Read the model definition and answer for the solid it produces. Units are mm, in the model's axes. A direction names the side the tool comes from. Coordinates: 2 decimals unless noted, no trailing zeros. Write each loop counter-clockwise with the first axis right and the second up, starting at its lowest first coordinate (ties: lowest second). Pieces come first, ordered by that corner, then holes. Notation, with made-up numbers: (22.5, 28) - (37.5, 28) arc R29 ccw to (37.5, 62) - close; hole circle Ø8 at (42, 13.25). An arc over 180 degrees is marked (long way). Return JSON: item names as keys, results as strings.
```python
from build123d import *

# Parameters (mm, degrees)
SKETCH001_R      = 16.5
SKETCH001_R_2    = 8
EXTRUDE001_DEPTH = 150
SKETCH002_R      = 10
SKETCH002_R_2    = 4
EXTRUDE002_DEPTH = 60
SKETCH003_W      = 50
SKETCH003_H      = 60
SKETCH003_R      = 3.25
EXTRUDE003_DEPTH = 7
SKETCH_R         = 25.4
SKETCH_R_2       = 15.875
EXTRUDE_DEPTH    = 50
FILLET_1_R       = 6
FILLET_2_R       = 4
FILLET_3_R       = 3
FILLET_4_R       = 2
FILLET_5_R       = 1.5


with BuildPart() as midpipe:
    # Sketch001 → Extrude001 (new body)
    with BuildSketch(Plane.XY):
        Circle(SKETCH001_R)
        Circle(SKETCH001_R_2, mode=Mode.SUBTRACT)
    extrude(amount=-EXTRUDE001_DEPTH)


with BuildPart() as basepipe:
    # Sketch002 → Extrude002 (new body)
    with BuildSketch(Plane.XY.offset(-150)):
        Circle(SKETCH002_R)
        Circle(SKETCH002_R_2, mode=Mode.SUBTRACT)
    extrude(amount=-EXTRUDE002_DEPTH)


with BuildPart() as obj1:
    # Sketch003 → Extrude003 (new body)
    with BuildSketch(Plane(origin=(0, 15, -185), x_dir=(1, 0, 0), z_dir=(0, -1, 0))):
        Rectangle(SKETCH003_W, SKETCH003_H)
        with Locations((-15, 12.75)):
            Circle(SKETCH003_R, mode=Mode.SUBTRACT)
        with Locations((-15, -3.25)):
            Circle(SKETCH003_R, mode=Mode.SUBTRACT)
        with Locations((15.5, 12.75)):
            Circle(SKETCH003_R, mode=Mode.SUBTRACT)
        with Locations((15.5, -3.250048)):
            Circle(SKETCH003_R, mode=Mode.SUBTRACT)
    extrude(amount=EXTRUDE003_DEPTH)


with BuildPart() as mountfillet:
    # Sketch → Extrude (new body)
    with BuildSketch(Plane.XY):
        Circle(SKETCH_R)
        Circle(SKETCH_R_2, mode=Mode.SUBTRACT)
    extrude(amount=EXTRUDE_DEPTH)

    # Fusion: union midPipe, basePipe, obj1
    add(midpipe.part)
    add(basepipe.part)
    add(obj1.part)

    # Fillet 1
    fillet_1_edges = [mountfillet.edges().sort_by_distance(p)[0] for p in [
        (-16.5, 0, 0),
    ]]
    fillet(fillet_1_edges, radius=FILLET_1_R)

    # Fillet 2
    fillet_2_edges = [mountfillet.edges().sort_by_distance(p)[0] for p in [
        (-10, 0, -150),
    ]]
    fillet(fillet_2_edges, radius=FILLET_2_R)

    # Fillet 3
    fillet_3_edges = [mountfillet.edges().sort_by_distance(p)[0] for p in [
        (6, 8, -182.5),
        (-6, 8, -182.5),
        (-25, 8, -185),
        (0, 8, -215),
        (25, 8, -185),
    ]]
    fillet(fillet_3_edges, radius=FILLET_3_R)

    # Fillet 4
    fillet_4_edges = [mountfillet.edges().sort_by_distance(p)[0] for p in [
        (-25.4, 0, 0),
    ]]
    fillet(fillet_4_edges, radius=FILLET_4_R)

    # Fillet 5
    fillet_5_edges = [mountfillet.edges().sort_by_distance(p)[0] for p in [
        (-16.5, 0, -150),
    ]]
    fillet(fillet_5_edges, radius=FILLET_5_R)


solid = mountfillet.part
```
(1) Flat-ended cylindrical pins translate along their axes: P1, Ø4.5, axis at y = 12.5, z = -178.5, coming from the -X side; P2, Ø2, axis at x = 8, y = -3.5, coming from the -Z side; P3, Ø4, axis at x = -2, y = 9.5, coming from the +Z side. Find the tip coordinate at first contact, or state that the pin passes through.
Answer:
{"P1": "x = -25", "P2": "z = -210", "P3": "z = 0"}
(2) A cutting plane is placed at B-B (z = -27.5). Determine the outline of the cut face in (x, y), and give its area (3 significant figures).
Answer:
{"outline": "circle Ø33 at (0, 0); hole circle Ø16 at (0, 0)", "area": "654 mm²"}
(3) Straight lines are drawn through the part: line 1 (X direction, y = 12, z = -172); line 2 (Z direction, x = -15, y = 9.5); line 3 (Z direction, x = 15.5, y = 11.5). For each, find the intervals that lie inside material, in ascending order. Write a range as from..to.
Answer:
{"line 1": "-25..-18.24, -11.76..12.26, 18.74..25", "line 2": "-214.6..-191.5, -185..-175.5, -169..-155, -2.33..50", "line 3": "-215..-191.5, -185..-175.5, -169..-155, -0.92..50"}
(4) Determine the mould class of faces 1 (the face through (-3, -3, -210)), 2 (the face through (-9.48, 6.63, -180.16)), 3 (the face through (-13.25, 11.55, -185.51)) for opening direction Z: +Z half, -Z half, draft (parallel to the pull), parting line (faces both ways), or undercut.
Answer:
{"face 1": "-Z half", "face 2": "draft", "face 3": "undercut"}
(5) A cutting plane is placed at C-C (z = 9.5). Determine the outline of the cut face in (x, y) (3 decimals), and give its area (3 significant figures).
Answer:
{"outline": "circle Ø50.8 at (0, 0); hole circle Ø31.75 at (0, 0)", "area": "1,240 mm²"}
(6) Which of the six approach directions +Z, -Z, +X, -X, +Y, -Y give full straight-line access (tool end or side, diameter ignored) to faces 4 (the face through (0, 12, -155)), 5 (the face through (-7.3, 3.8, 0)), 6 (the face through (-9.48, 6.63, -199.61)), 7 (the face through (15.24, -6.32, -76.25)), 8 (the face through (0, 15, -185))?
Answer:
{"face 4": "+Y", "face 5": "+Z", "face 6": "-Z, -X", "face 7": "none", "face 8": "-Z, +X, -X, +Y"}
